Geometry check sheet. Reference: drawing and pictorial views, mm from the part's lowest x, y, z. Round coordinates to 2 decimals unless told otherwise and drop trailing zeros. Write each loop counter-clockwise with the first axis right and the second up, starting at its lowest first coordinate (ties: lowest second). Pieces come first, ordered by that corner, then holes.
Item 1: Section check B-B, the plane z = 140. Record the cut outline in (x, y).
Item 2: Depth check by flat-ended pin: pin 1 (1.5 mm diameter, centred on y = 2, z = 67.5, fed in from -X); pin 2 (1.2 mm diameter, centred on x = 23, y = 2, fed in from -Z); pin 3 (1.2 mm diameter, centred on x = 20.5, y = 2.5, fed in from +Z). Enter the tip coordinate at first touch or a pass-through.
Item 3: Material ranges on line 1 along Z through (x, y) = (66.1, 2.85); line 2 along X through (y, z) = (2, 140); line 3 along X through (y, z) = (1.1, 53.5), recorded low to high.
Item 4: Section check C-C, the plane y = 1.7. State how many separate pieces and enclosed holes the cut face has, plus the area to 3 significant figures.
Item 5: Section check D-D, the plane z = 27. Record the cut outline in (x, y).
Item 6: Section check A-A, the plane x = 66.1. Record the cut outline in (y, z), plus the area to 3 significant figures.
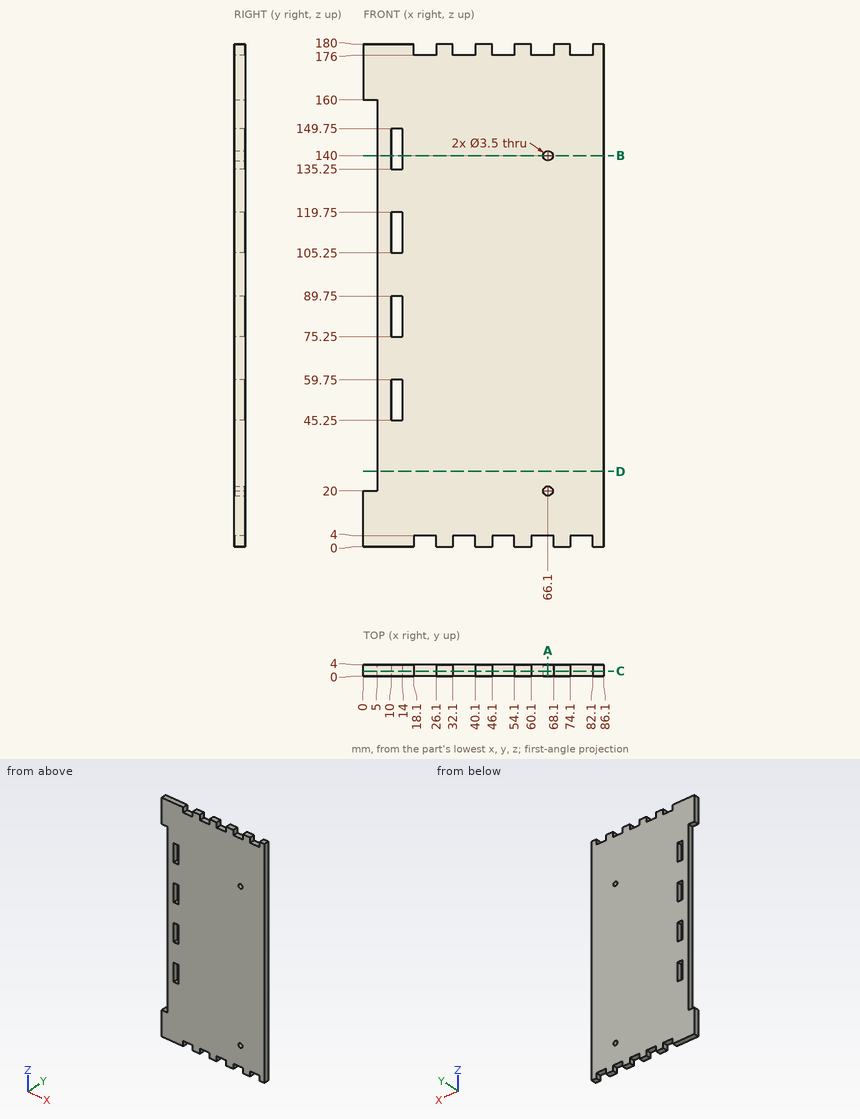
Values found:
1. outline: (5, 0) - (10, 0) - (10, 4) - (5, 4) - close; (14, 0) - (64.35, 0) - (64.35, 4) - (14, 4) - close; (67.85, 0) - (86.1, 0) - (86.1, 4) - (67.85, 4) - close
2. pin 1: stops at x = 5
2. pin 2: stops at z = 4
2. pin 3: stops at z = 176
3. line 1: z = 4 to 18.25, 21.75 to 138.25, 141.75 to 176
3. line 2: x = 5 to 10, 14 to 64.35, 67.85 to 86.1
3. line 3: x = 5 to 10, 14 to 86.1
4. separate pieces: 1
4. enclosed holes: 6
4. area: 14,200 mm2
5. outline: (5, 0) - (86.1, 0) - (86.1, 4) - (5, 4) - close
6. outline: (0, 4) - (4, 4) - (4, 18.25) - (0, 18.25) - close; (0, 21.75) - (4, 21.75) - (4, 138.25) - (0, 138.25) - close; (0, 141.75) - (4, 141.75) - (4, 176) - (0, 176) - close
6. area: 660 mm2
